```python
from build123d import *

# Parameters (mm, degrees)
F0_W     = 101.6
F0_H     = 50.8
F1_DEPTH = 457.2
F2_W     = 82.55
F2_H     = 31.75
F3_DEPTH = 457.2
F5_DEPTH = 101.6
F7_DEPTH = 101.6


with BuildPart() as f1:
    # F0 (on Top) → F1 (new body)
    with BuildSketch(Plane.XY):
        with Locations((50.8, 25.4)):
            Rectangle(F0_W, F0_H)
    extrude(amount=F1_DEPTH)

    # F2 (on face) → F3 (cut)
    with BuildSketch(Plane.XY.offset(457.2)):
        with Locations((50.8, 25.4)):
            Rectangle(F2_W, F2_H)
    extrude(amount=-F3_DEPTH, mode=Mode.SUBTRACT)

    # F4 (on face) → F5 (cut)
    with BuildSketch(Plane.YZ.offset(101.6)):
        Polygon((50.8, 50.8), (0, 0), (50.8, 0), align=None)
    extrude(amount=-F5_DEPTH, mode=Mode.SUBTRACT)

    # F6 (on face) → F7 (cut)
    with BuildSketch(Plane(origin=(0, 0, 0), x_dir=(0, -1, 0), z_dir=(-1, 0, 0))):
        Polygon((0, 457.2), (-50.8, 457.2), (-50.8, 406.4), align=None)
    extrude(amount=-F7_DEPTH, mode=Mode.SUBTRACT)


solid = f1.part
```
Can you work these out from the model? Positions are in its coordinate system, mm. A direction names the side the tool comes from. Coordinates: 2 decimals unless noted, no trailing zeros. Order: outer loops, then holes, each group sorted by start corner. A loop starts at its lowest first (then second) coordinate and runs counter-clockwise, first axis right, second up.
1. If we section it at B-B (y = 22.5): Please give me the cut outline in (x, z) (3 decimals).
2. Thinking about a two-plate mould opening in X: for faces 3 (the face through (50, 41.275, 231)), 4 (the face through (0, 25, 225)), 5 (the face through (101.6, 25, 225)), 6 (the face through (50, 50.8, 226)), which applies, +X half, -X half, draft (parallel to the pull), parting line (faces both ways), or undercut?
3. If we section it at C-C (z = 423.5): Please give me the cut outline in (x, y) (3 decimals).
4. For faces 1 (the face through (92.075, 25, 232)), 2 (the face through (50, 0, 225)), which set-ups out of +Z, -Z, +X, -X, +Y, -Y let a thin tool reach every point of the face, with its end or its side?
5. I need wall thicknesses on line 1 (X direction, y = 36.5, z = 246) (3 decimals); line 2 (Y direction, x = 28.5, z = 283.5) (3 decimals); line 3 (Y direction, x = 11, z = 419) (3 decimals). Which ranges of each line are inside material? Lowest first, please.
6. I'm going to push a flat-ended pin straight in: pin 1 (1.5 mm diameter, centred on x = 21.5, y = 8, fed in from -Z). Where does the tip first touch, or does it pass through?
7. If we section it at D-D (y = 46): Please give me the cut outline in (x, z).
8. If we section it at A-A (x = 19): Please give me the cut outline in (y, z) (3 decimals), then the cut area to 3 significant figures.
Entries:
1. outline: (0, 22.5) - (9.525, 22.5) - (9.525, 434.7) - (0, 434.7) - close; (92.075, 22.5) - (101.6, 22.5) - (101.6, 434.7) - (92.075, 434.7) - close
2. face 3: undercut
2. face 4: -X half
2. face 5: +X half
2. face 6: draft
3. outline: (0, 0) - (101.6, 0) - (101.6, 33.7) - (92.075, 33.7) - (92.075, 9.525) - (9.525, 9.525) - (9.525, 33.7) - (0, 33.7) - close
4. face 1: +Z, -Z
4. face 2: +Z, -Z, +X, -X, -Y
5. line 1: x = 0 to 9.525, 92.075 to 101.6
5. line 2: y = 0 to 9.525, 41.275 to 50.8
5. line 3: y = 0 to 9.525
6. pin 1: stops at z = 7.25
7. outline: (0, 46) - (101.6, 46) - (101.6, 411.2) - (0, 411.2) - close
8. outline: (0, 0) - (9.525, 9.525) - (9.525, 447.675) - (0, 457.2) - close; (41.275, 41.275) - (50.8, 50.8) - (50.8, 406.4) - (41.275, 415.925) - close
8. area: 7,740 mm2
